from build123d import *

# Parameters (mm, degrees)
SKETCH009_R   = 1.7
SKETCH009_R_2 = 2.1
PAD_DEPTH     = 3


with BuildPart() as part:
    # Sketch009 → Pad (new body)
    with BuildSketch(Plane.XY):
        with BuildLine():
            Line((-215, 219), (-4, 219))
            ThreePointArc((0, 215), (-1.171573, 217.828427), (-4, 219))
            Line((0, 215), (0, 4))
            ThreePointArc((-4, 0), (-1.171573, 1.171573), (0, 4))
            Line((-10, 0), (-4, 0))
            ThreePointArc((-12.360781, 1), (-11.281921, 0.260308), (-10, 0))
            Line((-27.817047, 16.957383), (-12.360781, 1))
            ThreePointArc((-27.817047, 16.957383), (-31.099605, 19.207981), (-35, 20))
            Line((-184, 20), (-35, 20))
            ThreePointArc((-184, 20), (-187.900395, 19.207981), (-191.182953, 16.957383))
            Line((-206.639219, 1), (-191.182953, 16.957383))
            ThreePointArc((-209, 0), (-207.718079, 0.260308), (-206.639219, 1))
            Line((-215, 0), (-209, 0))
            ThreePointArc((-219, 4), (-217.828427, 1.171573), (-215, 0))
            Line((-219, 215), (-219, 4))
            ThreePointArc((-215, 219), (-217.828427, 217.828427), (-219, 215))
        make_face()
        with Locations((-5, 214)):
            Circle(SKETCH009_R, mode=Mode.SUBTRACT)
        with Locations((-5, 109.5)):
            Circle(SKETCH009_R, mode=Mode.SUBTRACT)
        with Locations((-5, 5)):
            Circle(SKETCH009_R, mode=Mode.SUBTRACT)
        with Locations((-109.5, 214)):
            Circle(SKETCH009_R, mode=Mode.SUBTRACT)
        with Locations((-214, 214)):
            Circle(SKETCH009_R, mode=Mode.SUBTRACT)
        with Locations((-214, 5)):
            Circle(SKETCH009_R, mode=Mode.SUBTRACT)
        with Locations((-109.5, 130)):
            Circle(SKETCH009_R, mode=Mode.SUBTRACT)
        with Locations((-109.5, 89)):
            Circle(SKETCH009_R, mode=Mode.SUBTRACT)
        with Locations((-12.375, 83.3)):
            Circle(SKETCH009_R_2, mode=Mode.SUBTRACT)
        with Locations((-36.625, 83.3)):
            Circle(SKETCH009_R_2, mode=Mode.SUBTRACT)
        with Locations((-12.375, 74.3)):
            Circle(SKETCH009_R_2, mode=Mode.SUBTRACT)
        with Locations((-12.375, 65.3)):
            Circle(SKETCH009_R_2, mode=Mode.SUBTRACT)
        with Locations((-36.625, 74.3)):
            Circle(SKETCH009_R_2, mode=Mode.SUBTRACT)
        with Locations((-36.625, 65.3)):
            Circle(SKETCH009_R_2, mode=Mode.SUBTRACT)
        with Locations((-12.375, 154.7)):
            Circle(SKETCH009_R_2, mode=Mode.SUBTRACT)
        with Locations((-36.625, 154.7)):
            Circle(SKETCH009_R_2, mode=Mode.SUBTRACT)
        with Locations((-12.375, 145.7)):
            Circle(SKETCH009_R_2, mode=Mode.SUBTRACT)
        with Locations((-12.375, 136.7)):
            Circle(SKETCH009_R_2, mode=Mode.SUBTRACT)
        with Locations((-36.625, 145.7)):
            Circle(SKETCH009_R_2, mode=Mode.SUBTRACT)
        with Locations((-36.625, 136.7)):
            Circle(SKETCH009_R_2, mode=Mode.SUBTRACT)
        with Locations((-182.375, 83.3)):
            Circle(SKETCH009_R_2, mode=Mode.SUBTRACT)
        with Locations((-206.625, 83.3)):
            Circle(SKETCH009_R_2, mode=Mode.SUBTRACT)
        with Locations((-182.375, 74.3)):
            Circle(SKETCH009_R_2, mode=Mode.SUBTRACT)
        with Locations((-182.375, 65.3)):
            Circle(SKETCH009_R_2, mode=Mode.SUBTRACT)
        with Locations((-206.625, 74.3)):
            Circle(SKETCH009_R_2, mode=Mode.SUBTRACT)
        with Locations((-206.625, 65.3)):
            Circle(SKETCH009_R_2, mode=Mode.SUBTRACT)
        with Locations((-182.375, 154.7)):
            Circle(SKETCH009_R_2, mode=Mode.SUBTRACT)
        with Locations((-206.625, 154.7)):
            Circle(SKETCH009_R_2, mode=Mode.SUBTRACT)
        with Locations((-182.375, 145.7)):
            Circle(SKETCH009_R_2, mode=Mode.SUBTRACT)
        with Locations((-182.375, 136.7)):
            Circle(SKETCH009_R_2, mode=Mode.SUBTRACT)
        with Locations((-206.625, 145.7)):
            Circle(SKETCH009_R_2, mode=Mode.SUBTRACT)
        with Locations((-206.625, 136.7)):
            Circle(SKETCH009_R_2, mode=Mode.SUBTRACT)
        with Locations((-182.375, 119)):
            Circle(SKETCH009_R_2, mode=Mode.SUBTRACT)
        with Locations((-206.625, 119)):
            Circle(SKETCH009_R_2, mode=Mode.SUBTRACT)
        with Locations((-182.375, 110)):
            Circle(SKETCH009_R_2, mode=Mode.SUBTRACT)
        with Locations((-182.375, 101)):
            Circle(SKETCH009_R_2, mode=Mode.SUBTRACT)
        with Locations((-206.625, 110)):
            Circle(SKETCH009_R_2, mode=Mode.SUBTRACT)
        with Locations((-206.625, 101)):
            Circle(SKETCH009_R_2, mode=Mode.SUBTRACT)
        with BuildLine():
            Line((-27.625, 85.8), (-27.625, 61.8))
            ThreePointArc((-27.625, 61.8), (-27.478553, 61.446447), (-27.125, 61.3))
            Line((-27.125, 61.3), (-21.875, 61.3))
            ThreePointArc((-21.875, 61.3), (-21.521447, 61.446447), (-21.375, 61.8))
            Line((-21.375, 85.8), (-21.375, 61.8))
            ThreePointArc((-21.375, 85.8), (-21.521447, 86.153553), (-21.875, 86.3))
            Line((-27.125, 86.3), (-21.875, 86.3))
            ThreePointArc((-27.125, 86.3), (-27.478553, 86.153553), (-27.625, 85.8))
        make_face(mode=Mode.SUBTRACT)
        with BuildLine():
            Line((-90, 189), (-50, 189))
            ThreePointArc((-47.928932, 184), (-47.294019, 187.191922), (-50, 189))
            Line((-90, 141.928932), (-47.928932, 184))
            ThreePointArc((-95, 144), (-93.191922, 141.294019), (-90, 141.928932))
            Line((-95, 184), (-95, 144))
            ThreePointArc((-90, 189), (-93.535534, 187.535534), (-95, 184))
        make_face(mode=Mode.SUBTRACT)
        with BuildLine():
            Line((-170, 189), (-130, 189))
            ThreePointArc((-125, 184), (-126.464466, 187.535534), (-130, 189))
            Line((-125, 184), (-125, 144))
            ThreePointArc((-130, 141.928932), (-126.808078, 141.294019), (-125, 144))
            Line((-172.071068, 184), (-130, 141.928932))
            ThreePointArc((-170, 189), (-172.705981, 187.191922), (-172.071068, 184))
        make_face(mode=Mode.SUBTRACT)
        with BuildLine():
            Line((-95, 75), (-95, 45))
            ThreePointArc((-95, 45), (-93.535534, 41.464466), (-90, 40))
            Line((-90, 40), (-60, 40))
            ThreePointArc((-60, 40), (-57.294019, 41.808078), (-57.928932, 45))
            Line((-90, 77.071068), (-57.928932, 45))
            ThreePointArc((-90, 77.071068), (-93.191922, 77.705981), (-95, 75))
        make_face(mode=Mode.SUBTRACT)
        with BuildLine():
            Line((-162.071068, 45), (-130, 77.071068))
            ThreePointArc((-125, 75), (-126.808078, 77.705981), (-130, 77.071068))
            Line((-125, 75), (-125, 45))
            ThreePointArc((-130, 40), (-126.464466, 41.464466), (-125, 45))
            Line((-160, 40), (-130, 40))
            ThreePointArc((-162.071068, 45), (-162.705981, 41.808078), (-160, 40))
        make_face(mode=Mode.SUBTRACT)
        with BuildLine():
            Line((-27.625, 157.2), (-27.625, 133.2))
            ThreePointArc((-27.625, 133.2), (-27.478553, 132.846447), (-27.125, 132.7))
            Line((-27.125, 132.7), (-21.875, 132.7))
            ThreePointArc((-21.875, 132.7), (-21.521447, 132.846447), (-21.375, 133.2))
            Line((-21.375, 157.2), (-21.375, 133.2))
            ThreePointArc((-21.375, 157.2), (-21.521447, 157.553553), (-21.875, 157.7))
            Line((-27.125, 157.7), (-21.875, 157.7))
            ThreePointArc((-27.125, 157.7), (-27.478553, 157.553553), (-27.625, 157.2))
        make_face(mode=Mode.SUBTRACT)
        with BuildLine():
            Line((-197.625, 85.8), (-197.625, 61.8))
            ThreePointArc((-197.625, 61.8), (-197.478553, 61.446447), (-197.125, 61.3))
            Line((-197.125, 61.3), (-191.875, 61.3))
            ThreePointArc((-191.875, 61.3), (-191.521447, 61.446447), (-191.375, 61.8))
            Line((-191.375, 85.8), (-191.375, 61.8))
            ThreePointArc((-191.375, 85.8), (-191.521447, 86.153553), (-191.875, 86.3))
            Line((-197.125, 86.3), (-191.875, 86.3))
            ThreePointArc((-197.125, 86.3), (-197.478553, 86.153553), (-197.625, 85.8))
        make_face(mode=Mode.SUBTRACT)
        with BuildLine():
            Line((-197.625, 157.2), (-197.625, 133.2))
            ThreePointArc((-197.625, 133.2), (-197.478553, 132.846447), (-197.125, 132.7))
            Line((-197.125, 132.7), (-191.875, 132.7))
            ThreePointArc((-191.875, 132.7), (-191.521447, 132.846447), (-191.375, 133.2))
            Line((-191.375, 157.2), (-191.375, 133.2))
            ThreePointArc((-191.375, 157.2), (-191.521447, 157.553553), (-191.875, 157.7))
            Line((-197.125, 157.7), (-191.875, 157.7))
            ThreePointArc((-197.125, 157.7), (-197.478553, 157.553553), (-197.625, 157.2))
        make_face(mode=Mode.SUBTRACT)
        with BuildLine():
            Line((-197.625, 121.5), (-197.625, 97.5))
            ThreePointArc((-197.625, 97.5), (-197.478553, 97.146447), (-197.125, 97))
            Line((-197.125, 97), (-191.875, 97))
            ThreePointArc((-191.875, 97), (-191.521447, 97.146447), (-191.375, 97.5))
            Line((-191.375, 121.5), (-191.375, 97.5))
            ThreePointArc((-191.375, 121.5), (-191.521447, 121.853553), (-191.875, 122))
            Line((-197.125, 122), (-191.875, 122))
            ThreePointArc((-197.125, 122), (-197.478553, 121.853553), (-197.625, 121.5))
        make_face(mode=Mode.SUBTRACT)
    extrude(amount=PAD_DEPTH)


solid = part.part
Geometry: final body of the model. Coordinates: model frame, mm. A direction names the side the tool comes from. Coordinates: 2 decimals unless noted, no trailing zeros. Loops run counter-clockwise (first coordinate to the right, second up) from the corner with the lowest first, then second, coordinate; pieces in that order, holes last. Notation, with made-up numbers: (74.5, 63) - (124.5, 63) arc R24 cw to (124.5, 89) - close; hole circle Ø7 at (48, 74). An arc over 180 degrees is marked (long way). One line per question, with ' | ' between items. Start each with the question number.
(1) Draft query along Y for faces 4 (the flat face through (-199.019, 8.867, 1.479)), 5 (the cylindrical face through (-93, 188, 1)), 6 (the flat face through (-108, 111, 0)). Return one class per face: +Y half, -Y half, draft (parallel to the pull), parting line (faces both ways), or undercut.
(2) Cut plane A-A on x = -54. Output: boundary loops of the cut face in (y, z).
(3) Cut plane B-B on y = 165. Output: boundary loops of the cut face in (x, z), and give its area (3 significant figures).
(4) First-contact query: pin 1 (3.5 mm diameter, centred on x = -36.625, y = 154.7, fed in from -Z); pin 2 (0.9 mm diameter, centred on x = -154.5, z = 1, fed in from -Y). Flat tips, straight axial feed; report the tip coordinate or a pass-through.
(5) Reachability of faces 1 (the flat face through (-20.197, 9.09, 1.479)), 2 (the cylindrical face through (-94, 42, 1)), 3 (the flat face through (-108, 111, 3)) from +Z, -Z, +X, -X, +Y, -Y: full face, straight path, thin tool, end or side. Return the list, or none.
(6) Ray query, L1, parallel to X at y = 109.5, z = 2.2 (3 decimals); L2, parallel to X at y = 150, z = 1.6 (3 decimals); L3, parallel to Y at x = -85, z = 1.05. Return the intervals inside material, ascending. Write a range as from..to.
(7) Cut plane C-C on z = 0.55. Count the separate pieces of the cut face and the enclosed holes in it, and give its area (3 significant figures).
Here are the results:
1) face 4: -Y half | face 5: undercut | face 6: draft
2) outline: (20, 0) - (177.93, 0) - (177.93, 3) - (20, 3) - close; (189, 0) - (219, 0) - (219, 3) - (189, 3) - close
3) outline: (-219, 0) - (-153.07, 0) - (-153.07, 3) - (-219, 3) - close; (-125, 0) - (-95, 0) - (-95, 3) - (-125, 3) - close; (-66.93, 0) - (0, 0) - (0, 3) - (-66.93, 3) - close | area: 489 mm²
4) pin 1: through | pin 2: y = 20
5) face 1: +Z, -Z, -Y | face 2: +Z, -Z | face 3: +Z, +X, -X, +Y, -Y
6) L1: -219..-208.665, -204.585..-197.625, -191.375..-184.415, -180.335..-6.7, -3.3..0 | L2: -219..-197.625, -191.375..-138.071, -125..-95, -81.929..-27.625, -21.375..0 | L3: 20..40, 72.07..146.93, 189..219
7) separate pieces: 1 | enclosed holes: 47 | area: 38,800 mm²
